from build123d import *

# Parameters (mm, degrees)
EXTRUDE1_DEPTH           = 1.6
SKETCH4_W                = 9.5
SKETCH4_H                = 1.6
EXTRUDE2_DEPTH           = 25
SKETCH5_R                = 1.85
CUT_EXTRUDE1_DEPTH       = 87.666717949
CUT_EXTRUDE2_START       = -1.6
CUT_EXTRUDE2_OUTLINE_R   = 1.85
CUT_EXTRUDE2_OUTLINE_R_2 = 4
CUT_EXTRUDE2_DEPTH       = 1.6
FILLET1_R                = 2
FILLET2_R                = 2
FILLET3_R                = 2
FILLET4_R                = 2
FILLET5_R                = 2
FILLET6_R                = 2
FILLET7_R                = 2
FILLET8_R                = 2


# Read off the part's stored shape, not the designer's step: Cut-Extrude2
with BuildPart() as part:
    # Sketch1 → Extrude1 (new body)
    with BuildSketch(Plane(origin=(0, 0, 0), x_dir=(1, 0, 0), z_dir=(0, 1, 0))):
        Polygon((0, 0), (0, 53.2), (9.5, 53.2), (9.5, 48.6), (12.5, 48.6), (12.5, 56.6), (47.5, 56.6), (47.5, 48.6), (50.5, 48.6), (50.5, 53.2), (60, 53.2), (60, 0), (50.5, 0), (50.5, 4.6), (47.5, 4.6), (47.5, -3.4), (12.5, -3.4), (12.5, 4.6), (9.5, 4.6), (9.5, 0), align=None)
    extrude(amount=EXTRUDE1_DEPTH)

    # Sketch4 → Extrude2 (add)
    with BuildSketch(Plane(origin=(0, 1.6, 0), x_dir=(1, 0, 0), z_dir=(0, 1, 0))):
        with Locations((4.75, 52.4)):
            Rectangle(SKETCH4_W, SKETCH4_H)
        with Locations((55.25, 52.4)):
            Rectangle(SKETCH4_W, SKETCH4_H)
        with Locations((55.25, 0.8)):
            Rectangle(SKETCH4_W, SKETCH4_H)
        with Locations((4.75, 0.8)):
            Rectangle(SKETCH4_W, SKETCH4_H)
    extrude(amount=EXTRUDE2_DEPTH)

    # Sketch5 → Cut-Extrude1 (cut, through all)
    with BuildSketch(Plane.XY):
        with Locations((6.25, 21.6)):
            Circle(SKETCH5_R)
        with Locations((6.25, 11.6)):
            Circle(SKETCH5_R)
        with Locations((53.75, 21.6)):
            Circle(SKETCH5_R)
        with Locations((53.75, 11.6)):
            Circle(SKETCH5_R)
    extrude(amount=-CUT_EXTRUDE1_DEPTH, mode=Mode.SUBTRACT)

    # Cut-Extrude2 outline → Cut-Extrude2 (cut)
    with BuildSketch(Plane(origin=(0, 1.6, 0), x_dir=(1, 0, 0), z_dir=(0, 1, 0)).offset(CUT_EXTRUDE2_START)):
        with Locations((14, 10.6)):
            Circle(CUT_EXTRUDE2_OUTLINE_R)
        with Locations((14, 42.6)):
            Circle(CUT_EXTRUDE2_OUTLINE_R)
        with Locations((22, 42.6)):
            Circle(CUT_EXTRUDE2_OUTLINE_R_2)
        with Locations((30, 42.6)):
            Circle(CUT_EXTRUDE2_OUTLINE_R)
        with Locations((22, 34.6)):
            Circle(CUT_EXTRUDE2_OUTLINE_R)
        with Locations((22, 50.6)):
            Circle(CUT_EXTRUDE2_OUTLINE_R)
        with Locations((22, 10.6)):
            Circle(CUT_EXTRUDE2_OUTLINE_R_2)
        with Locations((30, 10.6)):
            Circle(CUT_EXTRUDE2_OUTLINE_R)
        with Locations((22, 2.6)):
            Circle(CUT_EXTRUDE2_OUTLINE_R)
        with Locations((22, 18.6)):
            Circle(CUT_EXTRUDE2_OUTLINE_R)
        with Locations((38, 10.6)):
            Circle(CUT_EXTRUDE2_OUTLINE_R_2)
        with Locations((46, 10.6)):
            Circle(CUT_EXTRUDE2_OUTLINE_R)
        with Locations((38, 2.6)):
            Circle(CUT_EXTRUDE2_OUTLINE_R)
        with Locations((38, 18.6)):
            Circle(CUT_EXTRUDE2_OUTLINE_R)
        with Locations((38, 42.6)):
            Circle(CUT_EXTRUDE2_OUTLINE_R_2)
        with Locations((46, 42.6)):
            Circle(CUT_EXTRUDE2_OUTLINE_R)
        with Locations((38, 34.6)):
            Circle(CUT_EXTRUDE2_OUTLINE_R)
        with Locations((38, 50.6)):
            Circle(CUT_EXTRUDE2_OUTLINE_R)
    extrude(amount=CUT_EXTRUDE2_DEPTH, mode=Mode.SUBTRACT)

    # Fillet1
    fillet1_edges = [part.edges().sort_by_distance(p)[0] for p in [
        (60, 26.6, -0.8),
    ]]
    fillet(fillet1_edges, radius=FILLET1_R)

    # Fillet2
    fillet2_edges = [part.edges().sort_by_distance(p)[0] for p in [
        (60, 26.6, -52.4),
        (9.5, 26.6, -52.4),
        (9.5, 26.6, -0.8),
    ]]
    fillet(fillet2_edges, radius=FILLET2_R)

    # Fillet3
    fillet3_edges = [part.edges().sort_by_distance(p)[0] for p in [
        (47.5, 0.8, 3.4),
    ]]
    fillet(fillet3_edges, radius=FILLET3_R)

    # Fillet4
    fillet4_edges = [part.edges().sort_by_distance(p)[0] for p in [
        (12.5, 0.8, 3.4),
        (50.5, 26.6, -0.8),
        (0, 26.6, -0.8),
        (0, 26.6, -52.4),
        (50.5, 26.6, -52.4),
    ]]
    fillet(fillet4_edges, radius=FILLET4_R)

    # Fillet5
    fillet5_edges = [part.edges().sort_by_distance(p)[0] for p in [
        (12.5, 0.8, -56.6),
    ]]
    fillet(fillet5_edges, radius=FILLET5_R)

    # Fillet6
    fillet6_edges = [part.edges().sort_by_distance(p)[0] for p in [
        (47.5, 0.8, -56.6),
    ]]
    fillet(fillet6_edges, radius=FILLET6_R)

    # Fillet7
    fillet7_edges = [part.edges().sort_by_distance(p)[0] for p in [
        (55.25, 0, 0),
        (4.75, 0, 0),
    ]]
    fillet(fillet7_edges, radius=FILLET7_R)

    # Fillet8
    fillet8_edges = [part.edges().sort_by_distance(p)[0] for p in [
        (4.75, 0, -53.2),
        (55.25, 0, -53.2),
    ]]
    fillet(fillet8_edges, radius=FILLET8_R)


solid = part.part
Work out the finished part from the listing and answer in its coordinate system (mm). A direction names the side the tool comes from. Give positions to 0.01 mm unless a question says otherwise; leave off trailing zeros. Loops run counter-clockwise (first coordinate to the right, second up) from the corner with the lowest first, then second, coordinate; pieces in that order, holes last. Notation, with made-up numbers: (19, 29) - (54, 29) arc R29 ccw to (54, 52) - close; hole circle Ø7 at (83, -27.5). An arc over 180 degrees is marked (long way). Answer in a Markdown table with one row per item.
(1) Section B-B (y = 6.25) is taken. Give the vertices of the cut face in (x, z).
Results list:
| item | result |
|---|---|
| outline | (0, -53.2) - (9.5, -53.2) - (9.5, -51.6) - (0, -51.6) - close; (0, -1.6) - (9.5, -1.6) - (9.5, 0) - (0, 0) - close; (50.5, -53.2) - (60, -53.2) - (60, -51.6) - (50.5, -51.6) - close; (50.5, -1.6) - (60, -1.6) - (60, 0) - (50.5, 0) - close |
(2) Section D-D (y = 21.6) is taken. State how many separate pieces and enclosed holes the cut face has, and give its area (3 significant figures).
Results list:
| item | result |
|---|---|
| separate pieces | 8 |
| enclosed holes | 0 |
| area | 37.1 mm² |
(3) For a pull along Y with two mould halves and no side action, classify faces 1 (the face through (8.93, 26, -0.81)), 2 (the face through (52.386, 12.85, -0.789)), 3 (the face through (36.532, 0.789, -17.474)), 4 (the face through (52.386, 22.85, -0.789)) as pulls with the +Y half, pulls with the -Y half, needs draft (parallel to the pull), parting line crosses it, or undercut.
Results list:
| item | result |
|---|---|
| face 1 | pulls with the +Y half |
| face 2 | undercut |
| face 3 | needs draft |
| face 4 | undercut |
(4) Section C-C (x = 38) is taken. Give the vertices of the cut face in (y, z).
Results list:
| item | result |
|---|---|
| outline | (0, -56.6) - (1.6, -56.6) - (1.6, -52.45) - (0, -52.45) - close; (0, -48.75) - (1.6, -48.75) - (1.6, -46.6) - (0, -46.6) - close; (0, -38.6) - (1.6, -38.6) - (1.6, -36.45) - (0, -36.45) - close; (0, -32.75) - (1.6, -32.75) - (1.6, -20.45) - (0, -20.45) - close; (0, -16.75) - (1.6, -16.75) - (1.6, -14.6) - (0, -14.6) - close; (0, -6.6) - (1.6, -6.6) - (1.6, -4.45) - (0, -4.45) - close; (0, -0.75) - (1.6, -0.75) - (1.6, 3.4) - (0, 3.4) - close |
(5) A tool of negligible diameter and unlimited length cuts with its end or side. For faces 5 (the face through (55.18, 0.57, -0.6)), 6 (the face through (4.4, 11.68, -52.39)), 7 (the face through (4.82, 0.57, -52.6)), 8 (the face through (51.07, 26, -52.41)), from which of +Z, -Z, +X, -X, +Y, -Y can it reach the whole face along a straight path? Write none if from no direction.
Results list:
| item | result |
|---|---|
| face 5 | +Z, +X, -Y |
| face 6 | +Z, -Z |
| face 7 | -Z, -X, -Y |
| face 8 | +Z, -Z, +Y |
(6) Flat-ended cylindrical pins translate along their axes: pin 1 Ø3 at (x, y) = (53.5, 9.5) entering from -Z; pin 2 Ø6 at (x, y) = (6.25, 11.6) entering from +Z; pin 3 Ø3.5 at (x, z) = (30, -42.6) entering from -Y; pin 4 Ø8 at (x, z) = (37.5, -32.5) entering from +Y. Find the tip coordinate at first contact, or state that the pin passes through.
Results list:
| item | result |
|---|---|
| pin 1 | stops at z = -53.2 |
| pin 2 | stops at z = 0 |
| pin 3 | passes through |
| pin 4 | stops at y = 1.6 |
(7) Consider L1, parallel to Z at x = 30, y = 0.7; L2, parallel to X at y = 0.4, z = -42.6; L3, parallel to Z at x = 4.5, y = 15.75. Determine where each line is inside the solid, lowest interval first. Write a range as [from, to].
Results list:
| item | result |
|---|---|
| L1 | z = [-56.6, -44.45], [-40.75, -12.45], [-8.75, 3.4] |
| L2 | x = [0, 12.15], [15.85, 18], [26, 28.15], [31.85, 34], [42, 44.15], [47.85, 60] |
| L3 | z = [-53.2, -51.6], [-1.6, 0] |
(8) Section A-A (x = 53.75) is taken. Give the vertices of the cut face in (y, z).
Results list:
| item | result |
|---|---|
| outline | (0, -51.2) arc R2 ccw to (2, -53.2) - (9.75, -53.2) - (9.75, -51.6) - (1.6, -51.6) - (1.6, -1.6) - (9.75, -1.6) - (9.75, 0) - (2, 0) arc R2 ccw to (0, -2) - close; (13.45, -53.2) - (19.75, -53.2) - (19.75, -51.6) - (13.45, -51.6) - close; (13.45, -1.6) - (19.75, -1.6) - (19.75, 0) - (13.45, 0) - close; (23.45, -53.2) - (26.6, -53.2) - (26.6, -51.6) - (23.45, -51.6) - close; (23.45, -1.6) - (26.6, -1.6) - (26.6, 0) - (23.45, 0) - close |
